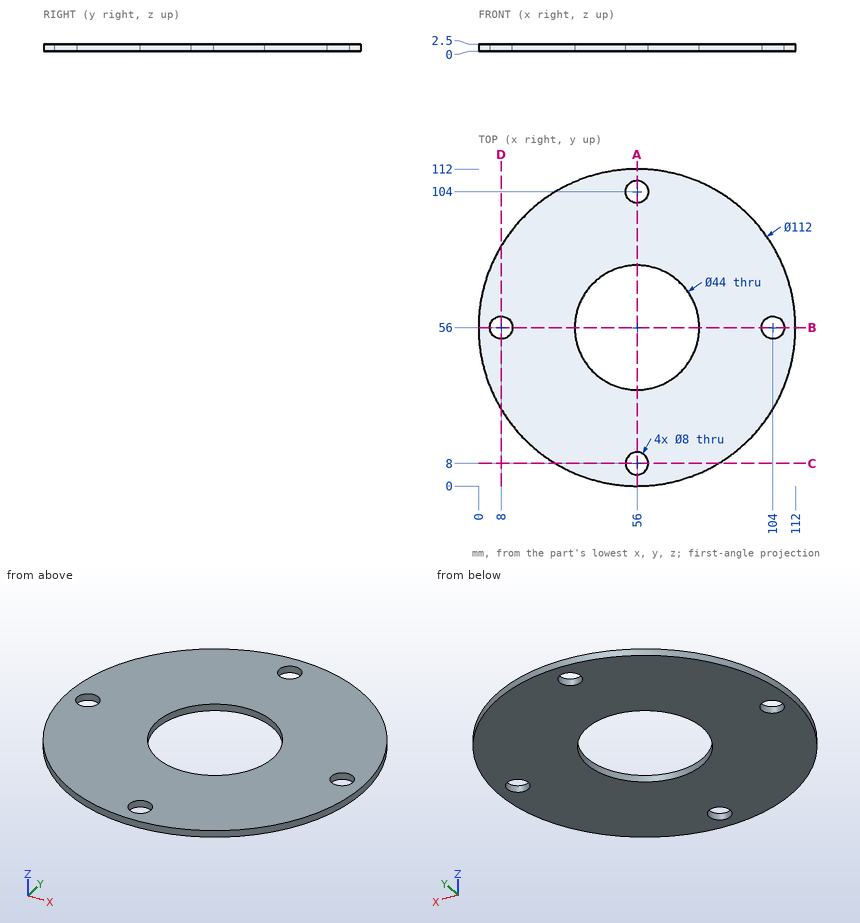
The drawing under review shows one solid part. Ordinate dimensions are in mm from its lowest x, y, z. Coordinates: 2 decimals unless noted, no trailing zeros. Order: outer loops, then holes, each group sorted by start corner. A loop starts at its lowest first (then second) coordinate and runs counter-clockwise, first axis right, second up. Notation, with made-up numbers: (-34, 74) -> (17, 74) arc R29 cw to (17, 108) -> close; hole circle Ø2 at (44, 44.25). An arc over 180 degrees is marked (long way). Answer in a Markdown table with one row per item. Add a question column.
Item 1: We need section A-A on x = 56. Write out the cut boundary in (y, z).
Item 2: To check wall thickness, follow probe 1 along Y at (x, z) = (56, 1.35); probe 2 along Y at (x, z) = (53, 2.3); probe 3 along Y at (x, z) = (104, 0.6). State the ranges of each line that lie inside material, in increasing order.
Item 3: We need section C-C on y = 8. Write out the cut boundary in (x, z).
Item 4: Clearance check with flat-ended pins moving along their axes: pin 1 (6.5 mm diameter, centred on x = 56, y = 104, fed in from +Z); pin 2 (1 mm diameter, centred on x = 19, z = 0.5, fed in from -Y). State where each tip first meets the part, or that it passes through.
Final values:
| question | item | result |
|---|---|---|
| 1 | outline | (0, 0) -> (4, 0) -> (4, 2.5) -> (0, 2.5) -> close; (12, 0) -> (34, 0) -> (34, 2.5) -> (12, 2.5) -> close; (78, 0) -> (100, 0) -> (100, 2.5) -> (78, 2.5) -> close; (108, 0) -> (112, 0) -> (112, 2.5) -> (108, 2.5) -> close |
| 2 | probe 1 | y = 0 to 4, 12 to 34, 78 to 100, 108 to 112 |
| 2 | probe 2 | y = 0.08 to 5.35, 10.65 to 34.21, 77.79 to 101.35, 106.65 to 111.92 |
| 2 | probe 3 | y = 27.16 to 52, 60 to 84.84 |
| 3 | outline | (27.16, 0) -> (52, 0) -> (52, 2.5) -> (27.16, 2.5) -> close; (60, 0) -> (84.84, 0) -> (84.84, 2.5) -> (60, 2.5) -> close |
| 4 | pin 1 | passes through |
| 4 | pin 2 | stops at y = 13.53 |
